```python
from build123d import *

# Parameters (mm, degrees)
EXTRUDE_1_DEPTH     = 3
EXTRUDE_1_TAPER     = 30
SKETCH_10_R         = 1
CUT_EXTRUDE_1_DEPTH = 10
CHAMFER_1_SIZE      = 2
EXTRUDE_2_DEPTH     = 1
EXTRUDE_2_TAPER     = 6
SKETCH_17_R         = 2.5
CUT_EXTRUDE_4_DEPTH = 2.4
CUT_EXTRUDE_2_DEPTH = 2
FILLET_1_R          = 1
SKETCH_13_R         = 2
CUT_EXTRUDE_3_DEPTH = 5220.265354769
SKETCH_14_R         = 14.5
EXTRUDE_3_DEPTH     = 3.2
FILLET_2_R          = 2


with BuildPart() as part:
    # Эскиз2 → Бобышка-Вытянуть1 (new body)
    with BuildSketch(Plane.XY):
        with BuildLine():
            ThreePointArc((4305.330098813, -2844.244902344), (4302.694059844, -2837.880941313), (4296.330098813, -2835.244902344))
            Line((4296.330098813, -2835.244902344), (4170.600097656, -2835.244902344))
            ThreePointArc((4170.600097656, -2835.244902344), (4164.236136626, -2837.880941313), (4161.600097656, -2844.244902344))
            Line((4161.600097656, -2844.244902344), (4161.600097656, -2941.399902344))
            ThreePointArc((4161.600097656, -2941.399902344), (4164.236136626, -2947.763863374), (4170.600097656, -2950.399902344))
            Line((4170.600097656, -2950.399902344), (4296.330098813, -2950.399902344))
            ThreePointArc((4296.330098813, -2950.399902344), (4302.694059844, -2947.763863374), (4305.330098813, -2941.399902344))
            Line((4305.330098813, -2941.399902344), (4305.330098813, -2844.244902344))
        make_face()
    extrude(amount=EXTRUDE_1_DEPTH, taper=EXTRUDE_1_TAPER)

    # Эскиз10 → Вырез-Вытянуть1 (cut)
    with BuildSketch(Plane.XY.offset(3)):
        with Locations((4167.600097656, -2841.244902344)):
            Circle(SKETCH_10_R)
        with Locations((4299.330098813, -2841.244902344)):
            Circle(SKETCH_10_R)
        with Locations((4167.600097656, -2944.399902344)):
            Circle(SKETCH_10_R)
        with Locations((4299.330098813, -2944.399902344)):
            Circle(SKETCH_10_R)
    extrude(amount=-CUT_EXTRUDE_1_DEPTH, mode=Mode.SUBTRACT)

    # Фаска1
    chamfer_1_edges = [part.edges().sort_by_distance(p)[0] for p in [
        (4298.330098813, -2841.244902344, 3),
        (4166.600097656, -2944.399902344, 3),
        (4298.330098813, -2944.399902344, 3),
        (4166.600097656, -2841.244902344, 3),
    ]]
    chamfer(chamfer_1_edges, length=CHAMFER_1_SIZE)

    # Эскиз11 → Бобышка-Вытянуть2 (add)
    with BuildSketch(Plane(origin=(0, 0, 0), x_dir=(-1, 0, 0), z_dir=(0, 0, -1))):
        with BuildLine():
            Line((-4301.330098813, -2846.244902344), (-4301.330098813, -2939.399902344))
            Line((-4301.330098813, -2939.399902344), (-4299.330098813, -2939.399902344))
            ThreePointArc((-4299.330098813, -2939.399902344), (-4295.794564907, -2940.864368438), (-4294.330098813, -2944.399902344))
            Line((-4294.330098813, -2944.399902344), (-4294.330098813, -2946.399902344))
            Line((-4294.330098813, -2946.399902344), (-4172.600097656, -2946.399902344))
            Line((-4172.600097656, -2946.399902344), (-4172.600097656, -2944.399902344))
            ThreePointArc((-4172.600097656, -2944.399902344), (-4171.135631562, -2940.864368438), (-4167.600097656, -2939.399902344))
            Line((-4167.600097656, -2939.399902344), (-4165.600097656, -2939.399902344))
            Line((-4165.600097656, -2939.399902344), (-4165.600097656, -2846.244902344))
            Line((-4165.600097656, -2846.244902344), (-4167.600097656, -2846.244902344))
            ThreePointArc((-4167.600097656, -2846.244902344), (-4171.135631562, -2844.78043625), (-4172.600097656, -2841.244902344))
            Line((-4172.600097656, -2841.244902344), (-4172.600097656, -2839.244902344))
            Line((-4172.600097656, -2839.244902344), (-4294.330098813, -2839.244902344))
            Line((-4294.330098813, -2839.244902344), (-4294.330098813, -2841.244902344))
            ThreePointArc((-4294.330098813, -2841.244902344), (-4295.794564907, -2844.78043625), (-4299.330098813, -2846.244902344))
            Line((-4299.330098813, -2846.244902344), (-4301.330098813, -2846.244902344))
        make_face()
    extrude(amount=EXTRUDE_2_DEPTH, taper=EXTRUDE_2_TAPER)

    # Эскиз17 → Вырез-Вытянуть4 (cut)
    with BuildSketch(Plane(origin=(0, 0, -1), x_dir=(-1, 0, 0), z_dir=(0, 0, -1))):
        with Locations((-4172.600097656, -2871.079902344)):
            Circle(SKETCH_17_R)
        with Locations((-4172.600097656, -2876.199902344)):
            Circle(SKETCH_17_R)
        with Locations((-4172.600097656, -2881.319902344)):
            Circle(SKETCH_17_R)
        with Locations((-4172.600097656, -2886.439902344)):
            Circle(SKETCH_17_R)
        with Locations((-4172.600097656, -2891.559902344)):
            Circle(SKETCH_17_R)
        with Locations((-4172.600097656, -2896.679902344)):
            Circle(SKETCH_17_R)
        with Locations((-4172.600097656, -2901.799902344)):
            Circle(SKETCH_17_R)
        with Locations((-4172.600097656, -2906.919902344)):
            Circle(SKETCH_17_R)
        with Locations((-4172.600097656, -2912.039902344)):
            Circle(SKETCH_17_R)
        with Locations((-4172.600097656, -2917.159902344)):
            Circle(SKETCH_17_R)
        with Locations((-4172.600097656, -2922.279902344)):
            Circle(SKETCH_17_R)
        with Locations((-4172.600097656, -2927.399902344)):
            Circle(SKETCH_17_R)
    extrude(amount=-CUT_EXTRUDE_4_DEPTH, mode=Mode.SUBTRACT)

    # Эскиз12 → Вырез-Вытянуть2 (cut)
    with BuildSketch(Plane.XY.offset(3)):
        with BuildLine():
            Line((4187.60009722, -2897.822402344), (4187.60009722, -2887.822402344))
            ThreePointArc((4187.60009722, -2887.822402344), (4195.60009722, -2879.822402344), (4203.60009722, -2887.822402344))
            Line((4203.60009722, -2887.822402344), (4203.60009722, -2897.822402344))
            ThreePointArc((4203.60009722, -2897.822402344), (4195.60009722, -2905.822402344), (4187.60009722, -2897.822402344))
        make_face()
    extrude(amount=-CUT_EXTRUDE_2_DEPTH, mode=Mode.SUBTRACT)

    # Скругление1
    fillet_1_edges = [part.edges().sort_by_distance(p)[0] for p in [
        (4195.60009722, -2905.822402344, 3),
        (4203.60009722, -2892.822402344, 3),
        (4195.60009722, -2879.822402344, 3),
        (4187.60009722, -2892.822402344, 3),
    ]]
    fillet(fillet_1_edges, radius=FILLET_1_R)

    # Эскиз13 → Вырез-Вытянуть3 (cut, through all)
    with BuildSketch(Plane.XY.offset(1)):
        with Locations((4195.60009722, -2892.822402344)):
            Circle(SKETCH_13_R)
    extrude(amount=-CUT_EXTRUDE_3_DEPTH, mode=Mode.SUBTRACT)

    # Эскиз14 → Бобышка-Вытянуть3 (add)
    with BuildSketch(Plane(origin=(0, 0, -1), x_dir=(-1, 0, 0), z_dir=(0, 0, -1))):
        with Locations((-4195.60009722, -2892.822402344)):
            Circle(SKETCH_14_R)
        Polygon((-4193.726947304, -2889.24125131), (-4197.764890032, -2889.409631415), (-4199.638039948, -2892.990782448), (-4197.473247136, -2896.403553377), (-4193.435304408, -2896.235173273), (-4191.562154492, -2892.654022239), align=None, mode=Mode.SUBTRACT)
    extrude(amount=EXTRUDE_3_DEPTH)

    # Скругление2
    fillet_2_edges = [part.edges().sort_by_distance(p)[0] for p in [
        (4210.10009722, -2892.822402344, -4.2),
    ]]
    fillet(fillet_2_edges, radius=FILLET_2_R)


solid = part.part
```
Build history of the part. All positions in model axes, mm. A direction names the side the tool comes from. Round coordinates to 2 decimals unless told otherwise and drop trailing zeros. Answer in a Markdown table with one row per item.
1) Pin check, flat tips, straight feed: P1, Ø1.5, axis at x = 4273.5, y = -2911.5, coming from the -Z side; P2, Ø3, axis at y = -2882.5, z = -1, coming from the -X side; P3, Ø2.5, axis at x = 4173.5, y = -2916.5, coming from the -Z side. Stop position of each tip, or through.
Values:
| item | result |
|---|---|
| P1 | z = -1 |
| P2 | x = 4161.6 |
| P3 | z = 1.4 |
2) Which spindle directions (+Z, -Z, +X, -X, +Y, -Y) get a long thin tool onto all of the face, cutting with end or side? Do faces 4 (the cylindrical face through (4195.78, -2905.82, 1.51)), 5 (the conical face through (4171.212, -2940.866, -0.507)), 6 (the flat face through (4173, -2886, 1.4)). Say none if no direction does.
Values:
| item | result |
|---|---|
| face 4 | +Z |
| face 5 | -Z, -X, -Y |
| face 6 | -Z |
3) Mould opens along Y. For faces 1 (the flat face through (4162.454, -2893.502, 1.479)), 2 (the flat face through (4173, -2922, 1.4)), 3 (the conical face through (4165.055, -2838.577, 1.854)) say: released by +Y, released by -Y, zero draft, split by the parting line, or undercut.
Values:
| item | result |
|---|---|
| face 1 | zero draft |
| face 2 | undercut |
| face 3 | released by +Y |
4) Wall check: L1, parallel to Z at x = 4299, y = -2890.5; L2, parallel to X at y = -2877, z = 0.25; L3, parallel to X at y = -2912, z = 0.75. Give the ranges that are in metal, low to high.
Values:
| item | result |
|---|---|
| L1 | -1 to 3 |
| L2 | 4161.74 to 4170.23, 4174.97 to 4305.19 |
| L3 | 4162.03 to 4170.1, 4175.1 to 4304.9 |
